For this review, take the finished solid that the model builds, in its own axes (mm). A direction names the side the tool comes from. Coordinates: 2 decimals unless noted, no trailing zeros. Order: outer loops, then holes, each group sorted by start corner. A loop starts at its lowest first (then second) coordinate and runs counter-clockwise, first axis right, second up. Notation, with made-up numbers: (21.5, -6.5) -> (77.5, -6.5) arc R18 cw to (77.5, -0.5) -> close; hole circle Ø10 at (-19.5, -21.5). An arc over 180 degrees is marked (long way). Write item = value, one per line. Start each with the question number.
1) Wall thickness on probe 1 along Y at (x, z) = (0, -0.75); probe 2 along X at (y, z) = (185, -5); probe 3 along Y at (x, z) = (-7.5, -17): over which ranges is each line inside the solid? List them lowest first. Write a range as [from, to].
2) Insertion check: pin 1 Ø9.5 at (y, z) = (-22.5, 3) entering from +X; pin 2 Ø9.5 at (y, z) = (183, -4) entering from -X; pin 3 Ø21 at (x, y) = (2, 179.5) entering from +Z; pin 4 Ø15 at (x, y) = (-1.5, 187.5) entering from -Z. Each pin has a flat end and moves straight along its axis. Give the tip position at first contact, or say it passes through.
3) Consider section B-B on x = 0. Give the boundary of the cut face in (y, z).
4) Consider section A-A on y = 185. Give the boundary of the cut face in (x, z), and give its area (3 significant figures).
5) Consider section D-D on z = -16.5. Give the boundary of the cut face in (x, y), and give its area (3 significant figures).
6) Draft analysis for pull direction Y (two halves, no side actions). For faces 1 (the face through (0, -30, 0)), 2 (the face through (9.5, 185, 0)), 3 (the face through (0.33, 187.48, -0.13)), state which applies: +Y half, -Y half, draft (parallel to the pull), parting line (faces both ways), or undercut.
7) Consider section C-C on x = -13. Give the boundary of the cut face in (y, z).
8) Machinability: for faces 4 (the face through (0, -11, -9.5)), 5 (the face through (0, 188, -9.5)), 6 (the face through (-9.5, 185, 0)), which of the approach directions +Z, -Z, +X, -X, +Y, -Y give a long, thin tool a straight path to every point of the face, cutting with its end or side? Answer none if there is none.
from build123d import *

# Parameters (mm, degrees)
SKETCH1_W           = 40
SKETCH1_H           = 40
BOSS_EXTRUDE1_DEPTH = 170
SKETCH2_W           = 19
SKETCH2_H           = 19
BOSS_EXTRUDE3_DEPTH = 30
SKETCH3_W           = 19
SKETCH3_H           = 19
BOSS_EXTRUDE4_DEPTH = 30
SKETCH4_R           = 2.5
CUT_EXTRUDE1_DEPTH  = 19


with BuildPart() as part:
    # Sketch1 → Boss-Extrude1 (new body)
    with BuildSketch(Plane(origin=(0, 0, 0), x_dir=(1, 0, 0), z_dir=(0, 1, 0))):
        Rectangle(SKETCH1_W, SKETCH1_H)
    extrude(amount=BOSS_EXTRUDE1_DEPTH)

    # Sketch2 → Boss-Extrude3 (add)
    with BuildSketch(Plane(origin=(0, 170, 0), x_dir=(1, 0, 0), z_dir=(0, 1, 0))):
        Rectangle(SKETCH2_W, SKETCH2_H)
    extrude(amount=BOSS_EXTRUDE3_DEPTH)

    # Sketch3 → Boss-Extrude4 (add)
    with BuildSketch(Plane.XZ):
        Rectangle(SKETCH3_W, SKETCH3_H)
    extrude(amount=BOSS_EXTRUDE4_DEPTH)

    # Sketch4 → Cut-Extrude1 (cut)
    with BuildSketch(Plane(origin=(0, 0, -9.5), x_dir=(-1, 0, 0), z_dir=(0, 0, -1))):
        with Locations((0, -15)):
            Circle(SKETCH4_R)
        with Locations((0, 185)):
            Circle(SKETCH4_R)
    extrude(amount=-CUT_EXTRUDE1_DEPTH, mode=Mode.SUBTRACT)


solid = part.part
Answer sheet:
q1.probe_1 = [-30, -17.5], [-12.5, 182.5], [187.5, 200]
q1.probe_2 = [-9.5, -2.5], [2.5, 9.5]
q1.probe_3 = [0, 170]
q2.pin_1 = 9.5
q2.pin_2 = -9.5
q2.pin_3 = 20
q2.pin_4 = -9.5
q3.outline = (-30, -9.5) -> (-17.5, -9.5) -> (-17.5, 9.5) -> (-30, 9.5) -> close; (-12.5, -9.5) -> (0, -9.5) -> (0, -20) -> (170, -20) -> (170, -9.5) -> (182.5, -9.5) -> (182.5, 9.5) -> (170, 9.5) -> (170, 20) -> (0, 20) -> (0, 9.5) -> (-12.5, 9.5) -> close; (187.5, -9.5) -> (200, -9.5) -> (200, 9.5) -> (187.5, 9.5) -> close
q4.outline = (-9.5, -9.5) -> (-2.5, -9.5) -> (-2.5, 9.5) -> (-9.5, 9.5) -> close; (2.5, -9.5) -> (9.5, -9.5) -> (9.5, 9.5) -> (2.5, 9.5) -> close
q4.area = 266 mm2
q5.outline = (-20, 0) -> (20, 0) -> (20, 170) -> (-20, 170) -> close
q5.area = 6,800 mm2
q6.face_1 = -Y half
q6.face_2 = draft
q6.face_3 = undercut
q7.outline = (0, -20) -> (170, -20) -> (170, 20) -> (0, 20) -> close
q8.face_4 = -Z, +X, -X, -Y
q8.face_5 = -Z, +X, -X, +Y
q8.face_6 = +Z, -Z, -X, +Y
